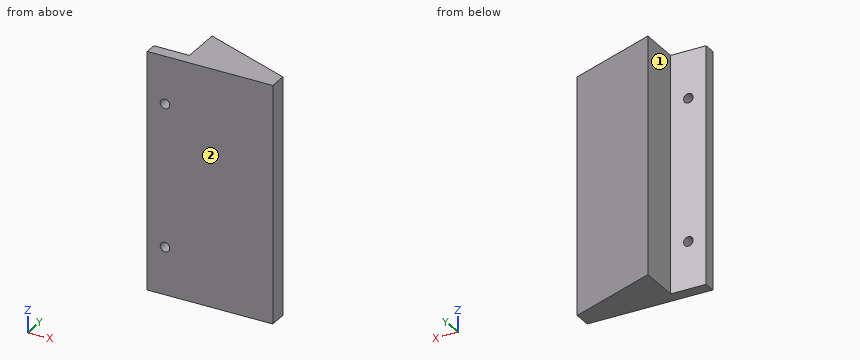
```python
from build123d import *

# Parameters (mm, degrees)
SALIENTE_EXTRUIR1_DEPTH = 100
CROQUIS2_R              = 2
CORTAR_EXTRUIR1_DEPTH   = 100


with BuildPart() as part:
    # Croquis1 → Saliente-Extruir1 (new body)
    with BuildSketch(Plane.XY):
        Polygon((0, 0), (-15, 0), (-15, 5), (0, 5), (0, 22), (38, 7.5), (38, 0), align=None)
    extrude(amount=SALIENTE_EXTRUIR1_DEPTH)

    # Croquis2 → Cortar-Extruir1 (cut)
    with BuildSketch(Plane(origin=(0, 5, 0), x_dir=(1, 0, 0), z_dir=(0, 1, 0))):
        with Locations((-7.5, -80)):
            Circle(CROQUIS2_R)
        with Locations((-7.5, -20)):
            Circle(CROQUIS2_R)
    extrude(amount=-CORTAR_EXTRUIR1_DEPTH, mode=Mode.SUBTRACT)


solid = part.part
```
The model under review builds one solid part; all positions refer to its coordinate system, in mm. Face numbers are marked on the shaded views. A direction names the side the tool comes from. Round coordinates to 2 decimals unless told otherwise and drop trailing zeros. Loops run counter-clockwise (first coordinate to the right, second up) from the corner with the lowest first, then second, coordinate; pieces in that order, holes last.
Item 1: Take a section at C-C (y = 6.5). Write out the cut boundary in (x, z), then the cut area to 3 significant figures.
Determined:
outline: (0, 0) - (38, 0) - (38, 100) - (0, 100) - close
area: 3,800 mm2
Item 2: For the marked faces 1 and 2, list the 3-axis set-ups (+Z, -Z, +X, -X, +Y, -Y) from which the entire face can be reached by the end or side of a thin tool; tool diameter is ignored.
Determined:
face 1: +Z, -Z, -X, +Y
face 2: +Z, -Z, +X, -X, -Y
Item 3: Take a section at D-D (x = 16). Write out the cut boundary in (y, z).
Determined:
outline: (0, 0) - (15.89, 0) - (15.89, 100) - (0, 100) - close
Item 4: Take a section at A-A (z = 20). Write out the cut boundary in (x, y), then the cut area to 4 significant figures.
Determined:
outline: (-15, 0) - (-9.5, 0) - (-9.5, 5) - (-15, 5) - close; (-5.5, 0) - (38, 0) - (38, 7.5) - (0, 22) - (0, 5) - (-5.5, 5) - close
area: 615.5 mm2
Item 5: Clearance check with flat-ended pins moving along their axes: pin 1 Ø2.5 at (x, z) = (-7.5, 80) entering from -Y; pin 2 Ø10 at (x, y) = (-4.5, 12) entering from -Z; pin 3 Ø8.5 at (y, z) = (14.5, 74) entering from -X; pin 4 Ø8 at (x, z) = (-8, 47) entering from +Y. State where each tip first meets the part, or that it passes through.
Determined:
pin 1: passes through
pin 2: stops at z = 0
pin 3: stops at x = 0
pin 4: stops at y = 5
Item 6: Take a section at B-B (z = 55). Write out the cut boundary in (x, y).
Determined:
outline: (-15, 0) - (38, 0) - (38, 7.5) - (0, 22) - (0, 5) - (-15, 5) - close
Item 7: For line 1 (Z direction, x = -7.5, y = 3.45); line 2 (X direction, y = 3.4, z = 20); line 3 (Y direction, x = -2, z = 77), list the stretches that pass through material, from the lowest coordinate up.
Determined:
line 1: z = 0 to 18, 22 to 78, 82 to 100
line 2: x = -15 to -9.5, -5.5 to 38
line 3: y = 0 to 5
